Work out the finished part from the listing and answer in its coordinate system (mm). A direction names the side the tool comes from. Round coordinates to 2 decimals unless told otherwise and drop trailing zeros. Write each loop counter-clockwise with the first axis right and the second up, starting at its lowest first coordinate (ties: lowest second). Pieces come first, ordered by that corner, then holes. Notation, with made-up numbers: M 46.25,88 L 74.25,88 A23 ccw 74.25,105 Z; hole C 54,-18.75 d4. An arc over 180 degrees is marked long. One line per item, written item: value. Start each with the question number.
Q1. Find section A-A (y = 5.25). Write down the section's boundary in (x, z).
Q2. Find section C-C (x = -29.5). Write down the section's boundary in (y, z).
Q3. The mould has two halves that part along X. Classify faces 1 (the cylindrical face through (-7.21, 1.48, -8.88)), 2 (the flat face through (-4, 6.15, 1)), 3 (the flat face through (10.28, 1.02, 1.02)): released by +X, released by -X, zero draft, split by the parting line, or undercut.
Q4. Find section D-D (x = -10). Write down the section's boundary in (y, z), and give its area (3 significant figures).
Q5. A tool of negligible diameter and unlimited length cuts with its end or side. For faces 4 (the flat face through (-0.69, 2, -24)), 5 (the flat face through (-0.69, 2, 27)), 6 (the flat face through (6, 2, -26.092)), 7 (the flat face through (-18.826, 1.479, -12.183)), from which of +Z, -Z, +X, -X, +Y, -Y can it reach the whole face along a straight path? Write none if from no direction.
Q6. Given pin 1 Ø5 at (x, z) = (-28.5, -3) entering from -Y; pin 2 Ø2.5 at (y, z) = (4.5, 22) entering from +X; pin 3 Ø2.5 at (y, z) = (2, -25) entering from -X; pin 4 Ø1 at (x, y) = (-11, 4) entering from +Z, each flat-ended and moving along its own axis, determine where each tip first touches the part or whether it passes through.
Q7. Consider probe 1 along Z at (x, y) = (-8, 1); probe 2 along X at (y, z) = (1.5, -5); probe 3 along X at (y, z) = (1.25, 8). Determine where each line is inside the solid, lowest interval first.
Q8. Find section B-B (z = 1). Write down the section's boundary in (x, y).
from build123d import *

# Parameters (mm, degrees)
BOSS_EXTRUDE1_DEPTH = 4
BOSS_EXTRUDE2_DEPTH = 2.25
SKETCH3_R           = 7.95
CUT_EXTRUDE1_DEPTH  = 9.25
SKETCH4_R           = 1.65
CUT_EXTRUDE2_DEPTH  = 9.25
CUT_EXTRUDE3_DEPTH  = 3
FILLET1_R           = 2.38125
CHAMFER1_SIZE       = 3.5
CHAMFER1_SIZE2      = 2.020725942
BOSS_EXTRUDE3_DEPTH = 4
SKETCH7_W           = 56.562445917
SKETCH7_H           = 51.963873078
CUT_EXTRUDE4_DEPTH  = 0.1
FILLET3_R           = 2.38


with BuildPart() as part:
    # Sketch1 → Boss-Extrude1 (new body)
    with BuildSketch(Plane(origin=(0, 0, 0), x_dir=(1, 0, 0), z_dir=(0, 1, 0))):
        with BuildLine():
            Line((-13.29118379, 20.889836125), (-0.68999579, 20.889836125))
            Line((-0.68999579, 20.889836125), (-0.68999579, 24.09210312))
            Line((-0.68999579, 24.09210312), (-0.68999579, 26.09210312))
            Line((-0.68999579, 26.09210312), (12.01000421, 26.09210312))
            Line((12.01000421, 26.09210312), (12.01000421, 24.09210312))
            Line((12.01000421, 24.09210312), (12.01000421, -26.90789688))
            Line((12.01000421, -26.90789688), (12.01000421, -28.90789688))
            Line((12.01000421, -28.90789688), (-0.68999579, -28.90789688))
            Line((-0.68999579, -28.90789688), (-0.68999579, -26.90789688))
            Line((-0.68999579, -26.90789688), (-0.68999579, -23.705629885))
            Line((-0.68999579, -23.705629885), (-13.29118379, -23.705629885))
            ThreePointArc((-13.29118379, -23.705629885), (-35.588916795, -1.40789688), (-13.29118379, 20.889836125))
        make_face()
    extrude(amount=BOSS_EXTRUDE1_DEPTH)

    # Sketch2 → Boss-Extrude2 (add)
    with BuildSketch(Plane(origin=(0, 4, 0), x_dir=(1, 0, 0), z_dir=(0, 1, 0))):
        with BuildLine():
            Line((-0.68999579, 20.889836125), (-0.68999579, 16.987726462))
            ThreePointArc((-0.68999579, 16.987726462), (9.006549215, -1.40789688), (-0.68999579, -19.803520222))
            Line((-0.68999579, -19.803520222), (-0.68999579, -23.705629885))
            Line((-0.68999579, -23.705629885), (-13.29118379, -23.705629885))
            ThreePointArc((-13.29118379, -23.705629885), (-35.588916795, -1.40789688), (-13.29118379, 20.889836125))
            Line((-13.29118379, 20.889836125), (-0.68999579, 20.889836125))
        make_face()
    extrude(amount=BOSS_EXTRUDE2_DEPTH)

    # Sketch3 → Cut-Extrude1 (cut)
    with BuildSketch(Plane.XZ):
        with Locations(Location((-13.29118379, 1.40789688, 0), (0, 0, 270))):
            Circle(SKETCH3_R)
    extrude(amount=-CUT_EXTRUDE1_DEPTH, mode=Mode.SUBTRACT)

    # Sketch4 → Cut-Extrude2 (cut)
    with BuildSketch(Plane.XZ):
        with Locations(Location((3.31000421, -21.59210312, 0), (0, 0, 270))):
            Circle(SKETCH4_R)
        with Locations(Location((3.31000421, 24.40789688, 0), (0, 0, 270))):
            Circle(SKETCH4_R)
    extrude(amount=-CUT_EXTRUDE2_DEPTH, mode=Mode.SUBTRACT)

    # Sketch5 → Cut-Extrude3 (cut)
    with BuildSketch(Plane.XZ):
        with BuildLine():
            ThreePointArc((-20.917233099, -7.792422241), (-25.24118379, 1.40789688), (-20.917233099, 10.608216001))
            Line((-20.917233099, 10.608216001), (-24.193916765, 16.291878661))
            ThreePointArc((-24.193916765, 16.291878661), (-31.74118379, 1.40789688), (-24.193916765, -13.476084902))
            Line((-24.193916765, -13.476084902), (-20.917233099, -7.792422241))
        make_face()
        with BuildLine():
            Line((-20.729723635, 18.291931497), (-17.445869217, 12.612408873))
            ThreePointArc((-17.445869217, 12.612408873), (-7.31618379, 11.756900455), (-1.510449053, 3.412089752))
            Line((-1.510449053, 3.412089752), (5.05008903, 3.407949716))
            ThreePointArc((5.05008903, 3.407949716), (-4.06618379, 17.38606558), (-20.729723635, 18.291931497))
        make_face()
        with BuildLine():
            ThreePointArc((-1.510449053, -0.596295992), (-7.31618379, -8.941106696), (-17.445869217, -9.796615113))
            Line((-17.445869217, -9.796615113), (-20.729723635, -15.476137738))
            ThreePointArc((-20.729723635, -15.476137738), (-4.06618379, -14.57027182), (5.05008903, -0.592155956))
            Line((5.05008903, -0.592155956), (-1.510449053, -0.596295992))
        make_face()
    extrude(amount=-CUT_EXTRUDE3_DEPTH, mode=Mode.SUBTRACT)

    # Fillet1
    fillet1_edges = [part.edges().sort_by_distance(p)[0] for p in [
        (-20.917233099, 1.5, 10.608216001),
        (-20.917233099, 1.5, -7.792422241),
        (-24.193916765, 1.5, -13.476084902),
        (-24.193916765, 1.5, 16.291878661),
        (5.05008903, 1.5, 3.407949716),
        (-1.510449053, 1.5, 3.412089752),
        (-17.445869217, 1.5, 12.612408873),
        (-20.729723635, 1.5, 18.291931497),
        (-17.445869217, 1.5, -9.796615113),
        (-1.510449053, 1.5, -0.596295992),
        (5.05008903, 1.5, -0.592155956),
        (-20.729723635, 1.5, -15.476137738),
    ]]
    fillet(fillet1_edges, radius=FILLET1_R)

    # Chamfer1
    chamfer1_edges = [part.edges().sort_by_distance(p)[0] for p in [
        (12.01000421, 0, 1.40789688),
    ]]
    chamfer1_side = [part.faces().sort_by_distance(p)[0] for p in [
        (-3.702499267, 0, 18.015985651),
    ]]
    chamfer(chamfer1_edges, length=CHAMFER1_SIZE, length2=CHAMFER1_SIZE2, reference=chamfer1_side[0])

    # Sketch6 → Boss-Extrude3 (add)
    with BuildSketch(Plane.XZ):
        with BuildLine():
            Line((-0.68999579, -22.889836125), (-13.29118379, -22.889836125))
            ThreePointArc((-13.29118379, -22.889836125), (-37.588916795, 1.40789688), (-13.29118379, 25.705629885))
            Line((-13.29118379, 25.705629885), (-0.68999579, 25.705629885))
            Line((-0.68999579, 25.705629885), (-0.68999579, 23.705629885))
            Line((-0.68999579, 23.705629885), (-13.29118379, 23.705629885))
            ThreePointArc((-13.29118379, 23.705629885), (-35.588916795, 1.40789688), (-13.29118379, -20.889836125))
            Line((-13.29118379, -20.889836125), (-0.68999579, -20.889836125))
            Line((-0.68999579, -20.889836125), (-0.68999579, -22.889836125))
        make_face()
    extrude(amount=-BOSS_EXTRUDE3_DEPTH)

    # Sketch7 → Cut-Extrude4 (cut)
    with BuildSketch(Plane(origin=(0, 6.25, 0), x_dir=(1, 0, 0), z_dir=(0, 1, 0))):
        with Locations((-12.789456293, -2.500057929)):
            Rectangle(SKETCH7_W, SKETCH7_H)
    extrude(amount=-CUT_EXTRUDE4_DEPTH, mode=Mode.SUBTRACT)

    # Fillet3
    fillet3_edges = [part.edges().sort_by_distance(p)[0] for p in [
        (-0.68999579, 5.075, -16.987726462),
        (-0.68999579, 5.075, 19.803520222),
    ]]
    fillet(fillet3_edges, radius=FILLET3_R)


solid = part.part
The answers:
1. outline: M -13.29,-20.89 L -0.69,-20.89 L -0.69,-18.2 A2.38 cw 0.25,-16.31 A22.3 ccw 0.25,19.13 A2.38 cw -0.69,21.02 L -0.69,23.71 L -13.29,23.71 A22.3 ccw Z; hole C -13.29,1.41 d15.9
2. outline: M 0,-16.69 L 4,-16.69 L 4,-13.9 L 6.15,-13.9 L 6.15,16.72 L 4,16.72 L 4,19.51 L 0,19.51 L 0,10.22 L 3,10.22 L 3,-7.41 L 0,-7.41 Z
3. face 1: undercut
3. face 2: zero draft
3. face 3: released by +X
4. outline: M 0,-22.89 L 4,-22.89 L 4,-20.89 L 6.15,-20.89 L 6.15,-5.83 L 0,-5.83 L 0,-10.08 L 3,-10.08 L 3,-16.75 L 0,-16.75 Z; M 0,8.64 L 6.15,8.64 L 6.15,23.71 L 4,23.71 L 4,25.71 L 0,25.71 L 0,19.56 L 3,19.56 L 3,12.9 L 0,12.9 Z
4. area: 161 mm2
5. face 4: -Z, -X, +Y, -Y
5. face 5: +Z, -X, +Y, -Y
5. face 6: -Z, +X, -X, +Y, -Y
5. face 7: -Y
6. pin 1: y = 3
6. pin 2: x = 12.01
6. pin 3: x = -0.69
6. pin 4: z = 25.71
7. probe 1: -22.89 to -16.27, -9.31 to -4.53, 7.34 to 12.12, 19.08 to 25.71
7. probe 2: -36.73 to -30.59, -23.38 to -18, -8.59 to -3.2, 4.01 to 11.11
7. probe 3: -36.68 to -30.52, -23.26 to -17.73, -8.85 to -3.32, 3.94 to 10.68
8. outline: M -37.59,0 L -31.74,0 L -31.74,3 L -25.23,3 L -25.23,0 L -21.23,0 L -21.23,6.15 L -35.59,6.15 L -35.59,4 L -37.59,4 Z; M -5.35,0 L 8.51,0 L 12.01,2.02 L 12.01,4 L 9,4 L 9,6.15 L -5.35,6.15 Z
